Input: dimensioned drawing with shaded views. Units: mm. Origin: part minimum x, y, z. A direction names the side the tool comes from. Coordinates: 2 decimals unless noted, no trailing zeros. Order: outer loops, then holes, each group sorted by start corner. A loop starts at its lowest first (then second) coordinate and runs counter-clockwise, first axis right, second up. Notation, with made-up numbers: (84.5, -35.75) - (135.5, -35.75) arc R6 ccw to (135.5, -27.75) - close; hole circle Ø1 at (65.5, 88.25). An arc over 180 degrees is marked (long way). One line per question, with ' | ' between items. Start each with the question number.
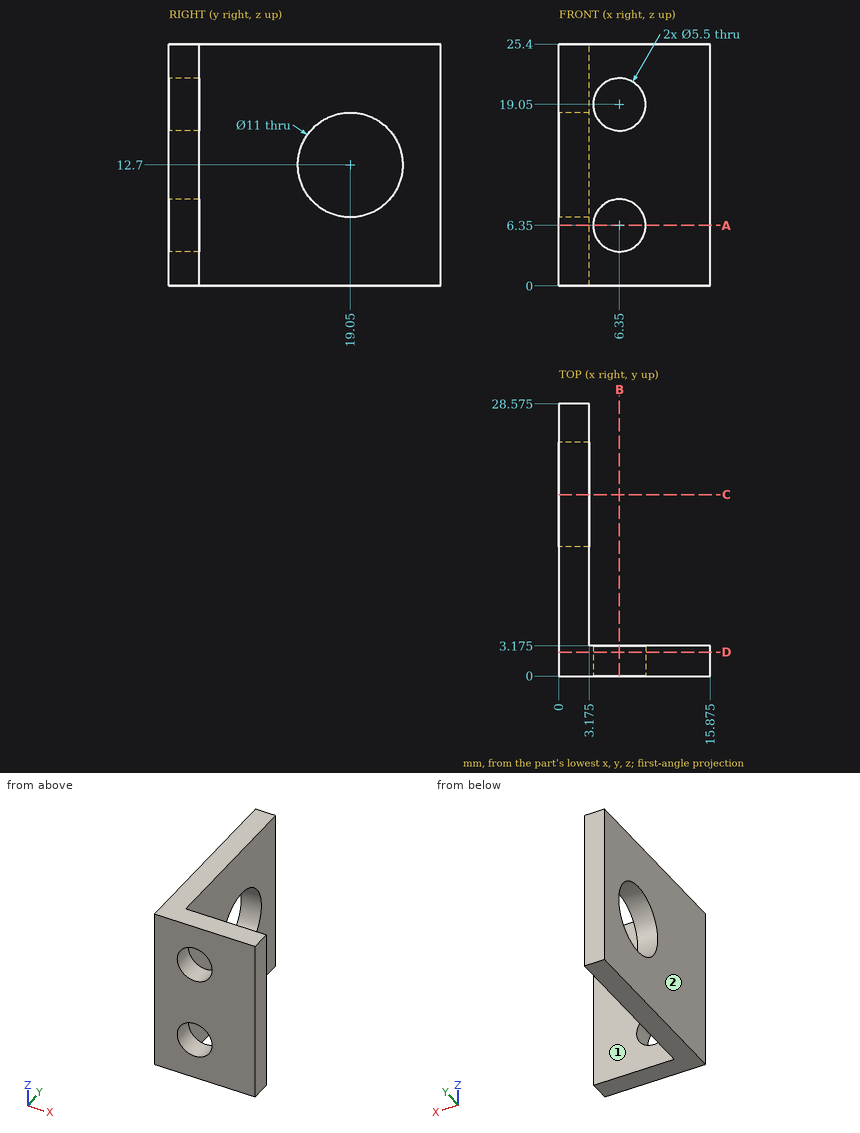
(1) Material intervals for line 1 along Z through (x, y) = (6.35, 1); line 2 along X through (y, z) = (1.55, 19.05) (3 decimals); line 3 along Y through (x, z) = (2.2, 12.7) (3 decimals), sorted ascending. Write a range as from..to.
(2) Section D-D (y = 2.5). Output: boundary loops of the cut face in (x, z) (3 decimals), then the cut area to 3 significant figures.
(3) Section C-C (y = 19.05). Output: boundary loops of the cut face in (x, z) (3 decimals).
(4) Section A-A (z = 6.35). Output: boundary loops of the cut face in (x, y) (3 decimals).
(5) Reachability of the marked faces 1 and 2 from +Z, -Z, +X, -X, +Y, -Y: full face, straight path, thin tool, end or side. Return the list, or none.
(6) Pin query (flat end, axial travel): pin 1 (4 mm diameter, centred on x = 7, z = 13, fed in from +Y) (3 decimals); pin 2 (12.5 mm diameter, centred on y = 19.5, z = 13, fed in from +X) (3 decimals). Return the tip coordinate at first contact, or that it passes through.
(7) Section B-B (x = 6.35). Output: boundary loops of the cut face in (y, z) (3 decimals), then the cut area to 3 significant figures.
Worked answers:
1) line 1: z = 0..3.6, 9.1..16.3, 21.8..25.4 | line 2: x = 0..3.6, 9.1..15.875 | line 3: y = 0..13.55, 24.55..28.575
2) outline: (0, 0) - (15.875, 0) - (15.875, 25.4) - (0, 25.4) - close; hole circle Ø5.5 at (6.35, 6.35); hole circle Ø5.5 at (6.35, 19.05) | area: 356 mm²
3) outline: (0, 0) - (3.175, 0) - (3.175, 7.2) - (0, 7.2) - close; (0, 18.2) - (3.175, 18.2) - (3.175, 25.4) - (0, 25.4) - close
4) outline: (0, 0) - (3.6, 0) - (3.6, 3.175) - (3.175, 3.175) - (3.175, 28.575) - (0, 28.575) - close; (9.1, 0) - (15.875, 0) - (15.875, 3.175) - (9.1, 3.175) - close
5) face 1: +Z, -Z, +X, +Y | face 2: +Z, -Z, -X, +Y, -Y
6) pin 1: stops at y = 3.175 | pin 2: stops at x = 3.175
7) outline: (0, 0) - (3.175, 0) - (3.175, 3.6) - (0, 3.6) - close; (0, 9.1) - (3.175, 9.1) - (3.175, 16.3) - (0, 16.3) - close; (0, 21.8) - (3.175, 21.8) - (3.175, 25.4) - (0, 25.4) - close | area: 45.7 mm²
